Work out the finished part from the listing and answer in its coordinate system (mm). A direction names the side the tool comes from. Give positions to 0.01 mm unless a question says otherwise; leave off trailing zeros. Order: outer loops, then holes, each group sorted by start corner. A loop starts at its lowest first (then second) coordinate and runs counter-clockwise, first axis right, second up. Notation, with made-up numbers: (0.5, 8.5) -> (48.5, 8.5) arc R25 ccw to (48.5, 47.5) -> close; hole circle Ø5 at (-26.5, -8.75). An arc over 180 degrees is marked (long way). Answer as CSV lines item,"result". Start each with the question number.
1. For faces 1 (the cylindrical face through (6.98, 0.1, 2.49)), 2 (the cylindrical face through (-0.86, -3.874, 0.783)), determine the directions among +Z, -Z, +X, -X, +Y, -Y from which every point of the face is accessible in a straight line to the end or side of a thin tool.
2. For a pull along X with two mould halves and no side action, classify faces 3 (the flat face through (-4.3, 0.1, 1.588)), 4 (the cylindrical face through (-15.714, -6.461, 2.348)), 5 (the flat face through (16.669, 0, 2)) as released by +X, released by -X, zero draft, split by the parting line, or undercut.
3. Find the intervals of material crossed by L1, parallel to X at y = -4, z = 3.45; L2, parallel to Y at x = 0, z = 0.7; L3, parallel to X at y = -2.75, z = 2, in increasing order.
4. Flat-ended cylindrical pins translate along their axes: pin 1 (1.3 mm diameter, centred on x = 13.589, y = -3.175, fed in from +Z); pin 2 (1.5 mm diameter, centred on x = 3.5, y = -5, fed in from +Z). Find the tip coordinate at first contact, or state that the pin passes through.
5. A cutting plane is placed at A-A (z = 2.7). State how many separate pieces and enclosed holes the cut face has, then the cut area to 3 significant figures.
6. A cutting plane is placed at B-B (x = 0). Give the vertices of the cut face in (y, z), then the cut area to 3 significant figures.
from build123d import *

# Parameters (mm, degrees)
SKETCH1_W          = 33.3375
SKETCH1_H          = 14.732
SKETCH1_R          = 3.96875
EXTRUDE1_DEPTH     = 1.5875
SKETCH3_W          = 8.73125
SKETCH3_H          = 14.732
EXTRUDE2_DEPTH     = 3.175
CUT_EXTRUDE1_START = -4.7625
SKETCH2_R          = 1.0795
SKETCH2_R_2        = 5.55625
CUT_EXTRUDE1_DEPTH = 4.7625
FILLET2_R          = 3.175
SPLIT1_DEPTH       = 4.7625


# Read off the part's stored shape, not the designer's step: Split1
with BuildPart() as part:
    # Sketch1 → Extrude1 (new body)
    with BuildSketch(Plane.XY):
        Rectangle(SKETCH1_W, SKETCH1_H)
        Circle(SKETCH1_R, mode=Mode.SUBTRACT)
    extrude(amount=EXTRUDE1_DEPTH)

    # Sketch3 → Extrude2 (add)
    with BuildSketch(Plane.XY.offset(1.5875)):
        with Locations((-12.303125, 0)):
            Rectangle(SKETCH3_W, SKETCH3_H)
        with Locations((12.303125, 0)):
            Rectangle(SKETCH3_W, SKETCH3_H)
    extrude(amount=EXTRUDE2_DEPTH)

    # Sketch2 → Cut-Extrude1 (cut)
    with BuildSketch(Plane(origin=(0, 0, 0), x_dir=(-1, 0, 0), z_dir=(0, 0, -1)).offset(CUT_EXTRUDE1_START)):
        with Locations((-13.589, -3.175)):
            Circle(SKETCH2_R)
        with Locations((13.589, 3.175)):
            Circle(SKETCH2_R)
        with Locations((0, 11.9126)):
            Circle(SKETCH2_R_2)
    extrude(amount=CUT_EXTRUDE1_DEPTH, mode=Mode.SUBTRACT)

    # Fillet2
    fillet2_edges = [part.edges().sort_by_distance(p)[0] for p in [
        (-7.9375, 0, 1.5875),
        (7.9375, 0, 1.5875),
    ]]
    fillet(fillet2_edges, radius=FILLET2_R - 0.0001)  # a hair under: the kernel refuses the full size

    # Split1 outline → Split1 (cut)
    with BuildSketch(Plane.XY):
        with BuildLine():
            Line((-16.66875, -7.366), (-13.49375, -7.366))
            ThreePointArc((-13.49375, -7.366), (-15.73881403, -6.43606403), (-16.66875, -4.191))
            Line((-16.66875, -4.191), (-16.66875, -7.366))
        make_face()
        with BuildLine():
            ThreePointArc((13.49375, 7.366), (15.73881403, 6.43606403), (16.66875, 4.191))
            Line((16.66875, 4.191), (16.66875, 7.366))
            Line((16.66875, 7.366), (13.49375, 7.366))
        make_face()
        with BuildLine():
            ThreePointArc((16.66875, -4.191), (15.73881403, -6.43606403), (13.49375, -7.366))
            Line((13.49375, -7.366), (16.66875, -7.366))
            Line((16.66875, -7.366), (16.66875, -4.191))
        make_face()
        with BuildLine():
            Line((-16.66875, 7.366), (-16.66875, 4.191))
            ThreePointArc((-16.66875, 4.191), (-15.73881403, 6.43606403), (-13.49375, 7.366))
            Line((-13.49375, 7.366), (-16.66875, 7.366))
        make_face()
    extrude(amount=SPLIT1_DEPTH, mode=Mode.SUBTRACT)


solid = part.part
Answer sheet:
1,face 1,"+Z, +Y, -Y"
1,face 2,"+Z, -Z"
2,face 3,"undercut"
2,face 4,"released by -X"
2,face 5,"released by +X"
3,L1,"x = -16.67 to -7.65, 7.65 to 12.89, 14.29 to 16.67"
3,L2,"y = -7.37 to -3.97, 3.97 to 6.36"
3,L3,"x = -16.67 to -6.33, 6.33 to 12.6, 14.58 to 16.67"
4,pin 1,"passes through"
4,pin 2,"stops at z = 1.59"
5,separate pieces,"2"
5,enclosed holes,"2"
5,area,"264 mm^2"
6,outline,"(-7.37, 0) -> (-3.97, 0) -> (-3.97, 1.59) -> (-7.37, 1.59) -> close; (3.97, 0) -> (6.36, 0) -> (6.36, 1.59) -> (3.97, 1.59) -> close"
6,area,"9.18 mm^2"
